```python
from build123d import *

# Parameters (mm, degrees)
SKETCH_1_R      = 1.75
SKETCH_1_R_2    = 1.55
SKETCH_1_W      = 10.25
SKETCH_1_H      = 4.9
EXTRUDE_1_DEPTH = 4
FILLET_1_R      = 1


with BuildPart() as part:
    # 草图1 → 凸台-拉伸1 (new body)
    with BuildSketch(Plane.XY):
        Polygon((-17.225, -19.5), (17.225, -19.5), (17.225, 19.5), (-14.225, 19.5), (-24.725, 19.5), (-24.725, 10.25), (-23.475, 9), (-23.475, 1), (-24.725, -0.25), (-24.725, -8), align=None)
        with BuildLine():
            Line((-5.775, -15.45), (-9.775, -15.45))
            ThreePointArc((-9.775, -15.45), (-10.825, -16.5), (-11.875, -15.45))
            Line((-11.875, -15.45), (-11.875, -12.4))
            ThreePointArc((-11.875, -12.4), (-10.825, -11.35), (-9.775, -12.4))
            Line((-9.775, -12.4), (-5.775, -12.4))
            ThreePointArc((-5.775, -12.4), (-4.725, -11.35), (-3.675, -12.4))
            Line((-3.675, -12.4), (-3.675, -15.45))
            ThreePointArc((-3.675, -15.45), (-4.725, -16.5), (-5.775, -15.45))
        make_face(mode=Mode.SUBTRACT)
        with Locations((-15.725, -7.5)):
            Circle(SKETCH_1_R, mode=Mode.SUBTRACT)
        with Locations((-21.225, -4)):
            Circle(SKETCH_1_R_2, mode=Mode.SUBTRACT)
        Polygon((-3.025, -8.4), (-12.225, -8.4), (-12.725, -8.4), (-12.725, -3.5), (-12.225, -3.5), (-3.025, -3.5), align=None, mode=Mode.SUBTRACT)
        with BuildLine():
            ThreePointArc((6.225, -15.45), (5.175, -16.5), (4.125, -15.45))
            Line((4.125, -15.45), (4.125, -12.4))
            ThreePointArc((4.125, -12.4), (5.175, -11.35), (6.225, -12.4))
            Line((6.225, -12.4), (10.225, -12.4))
            ThreePointArc((10.225, -12.4), (11.275, -11.35), (12.325, -12.4))
            Line((12.325, -12.4), (12.325, -15.45))
            ThreePointArc((12.325, -15.45), (11.275, -16.5), (10.225, -15.45))
            Line((10.225, -15.45), (6.225, -15.45))
        make_face(mode=Mode.SUBTRACT)
        with Locations((7.1, -5.95)):
            Rectangle(SKETCH_1_W, SKETCH_1_H, mode=Mode.SUBTRACT)
        with Locations((-15.725, 7.5)):
            Circle(SKETCH_1_R, mode=Mode.SUBTRACT)
        with Locations((-7.775, 0)):
            Circle(SKETCH_1_R_2, mode=Mode.SUBTRACT)
        Polygon((-12.225, 8.4), (-3.025, 8.4), (-3.025, 3.5), (-12.225, 3.5), (-12.725, 3.5), (-12.725, 8.4), align=None, mode=Mode.SUBTRACT)
        with Locations((-21.225, 14)):
            Circle(SKETCH_1_R_2, mode=Mode.SUBTRACT)
        with BuildLine():
            Line((-5.775, 12.4), (-9.775, 12.4))
            ThreePointArc((-9.775, 12.4), (-10.825, 11.35), (-11.875, 12.4))
            Line((-11.875, 12.4), (-11.875, 15.45))
            ThreePointArc((-11.875, 15.45), (-10.825, 16.5), (-9.775, 15.45))
            Line((-9.775, 15.45), (-5.775, 15.45))
            ThreePointArc((-5.775, 15.45), (-4.725, 16.5), (-3.675, 15.45))
            Line((-3.675, 15.45), (-3.675, 12.4))
            ThreePointArc((-3.675, 12.4), (-4.725, 11.35), (-5.775, 12.4))
        make_face(mode=Mode.SUBTRACT)
        with Locations((6.225, 0)):
            Circle(SKETCH_1_R_2, mode=Mode.SUBTRACT)
        with Locations((7.1, 5.95)):
            Rectangle(SKETCH_1_W, SKETCH_1_H, mode=Mode.SUBTRACT)
        with BuildLine():
            Line((10.225, 12.4), (6.225, 12.4))
            ThreePointArc((6.225, 12.4), (5.175, 11.35), (4.125, 12.4))
            Line((4.125, 12.4), (4.125, 15.45))
            ThreePointArc((4.125, 15.45), (5.175, 16.5), (6.225, 15.45))
            Line((6.225, 15.45), (10.225, 15.45))
            ThreePointArc((10.225, 15.45), (11.275, 16.5), (12.325, 15.45))
            Line((12.325, 15.45), (12.325, 12.4))
            ThreePointArc((12.325, 12.4), (11.275, 11.35), (10.225, 12.4))
        make_face(mode=Mode.SUBTRACT)
    extrude(amount=EXTRUDE_1_DEPTH)

    # 圆角1
    fillet_1_edges = [part.edges().sort_by_distance(p)[0] for p in [
        (-23.475, 1, 2),
        (-23.475, 9, 2),
        (-24.725, 10.25, 2),
        (-24.725, 19.5, 2),
        (17.225, 19.5, 2),
        (17.225, -19.5, 2),
        (-17.225, -19.5, 2),
        (-24.725, -8, 2),
        (-24.725, -0.25, 2),
        (-3.025, -8.4, 2),
        (-3.025, -3.5, 2),
        (-12.725, -3.5, 2),
        (-12.725, -8.4, 2),
        (-3.025, 3.5, 2),
        (-3.025, 8.4, 2),
        (-12.725, 8.4, 2),
        (-12.725, 3.5, 2),
        (12.225, 8.4, 2),
        (1.975, 8.4, 2),
        (1.975, 3.5, 2),
        (12.225, 3.5, 2),
        (1.975, -8.4, 2),
        (12.225, -8.4, 2),
        (12.225, -3.5, 2),
        (1.975, -3.5, 2),
    ]]
    fillet(fillet_1_edges, radius=FILLET_1_R)


solid = part.part
```
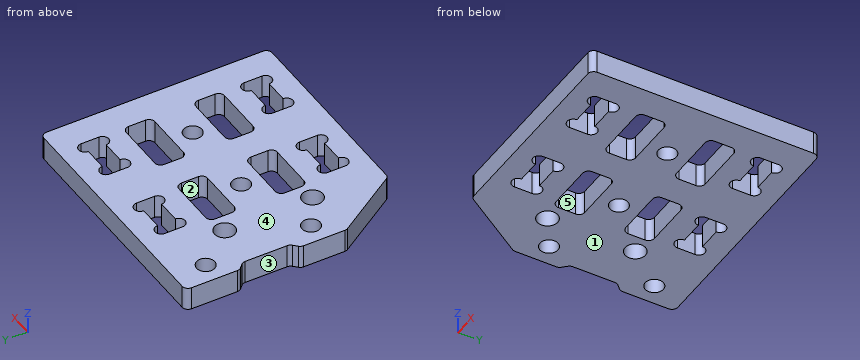
Can you work these out from the model? Positions are in its coordinate system, mm. Face numbers are marked on the shaded views. A direction names the side the tool comes from. Coordinates: 2 decimals unless noted, no trailing zeros. Write each loop counter-clockwise with the first axis right and the second up, starting at its lowest first coordinate (ties: lowest second). Pieces come first, ordered by that corner, then holes. Notation, with made-up numbers: (5.25, -30.75) - (19.25, -30.75) arc R20 ccw to (19.25, -6.75) - close; hole circle Ø9 at (61, 40). An arc over 180 degrees is marked (long way). Return JSON: item names as keys, results as strings.
Q1. Thinking about a two-plate mould opening in Y: for the marked faces 1 and 2, which applies, +Y half, -Y half, draft (parallel to the pull), parting line (faces both ways), or undercut?
Computed values:
{"face 1": "draft", "face 2": "undercut"}
Q2. I'm going to push flat-ended pins straight in: pin 1 Ø1.2 at (y, z) = (4.5, 2.5) entering from -X (3 decimals); pin 2 Ø4 at (x, y) = (-11.5, 9) entering from -Z; pin 3 Ø2 at (x, y) = (10, 13.5) entering from -Z. Where does each tip first touch, or does it pass through?
Computed values:
{"pin 1": "stops at x = -23.475", "pin 2": "stops at z = 0", "pin 3": "passes through"}
Q3. If we section it at A-A (y = -4): Please give me the cut outline in (x, z) (3 decimals), then the cut area to 3 significant figures.
Computed values:
{"outline": "(-24.725, 0) - (-22.775, 0) - (-22.775, 4) - (-24.725, 4) - close; (-19.675, 0) - (-12.591, 0) - (-12.591, 4) - (-19.675, 4) - close; (-3.159, 0) - (2.109, 0) - (2.109, 4) - (-3.159, 4) - close; (12.091, 0) - (17.225, 0) - (17.225, 4) - (12.091, 4) - close", "area": "77.7 mm2"}
Q4. On a 3-axis mill with a long thin cutter (end or side, diameter ignored), from which of +Z, -Z, +X, -X, +Y, -Y can I reach the whole of each face in a straight line? I mean the marked faces 3, 4 and 5. Say none if no direction works.
Computed values:
{"face 3": "+Z, -Z, -X", "face 4": "+Z, +X, -X, +Y, -Y", "face 5": "+Z, -Z"}
Q5. Please list where these lines run through material, in increasing order: L1, parallel to Y at x = 9, z = 2; L2, parallel to X at y = 5, z = 3.7 (3 decimals); L3, parallel to X at y = 4, z = 0.4 (3 decimals). Write a range as from..to.
Computed values:
{"L1": "y = -19.5..-15.45, -12.4..-8.4, -3.5..3.5, 8.4..12.4, 15.45..19.5", "L2": "x = -23.475..-12.725, -3.025..1.975, 12.225..17.225", "L3": "x = -23.475..-12.591, -3.159..2.109, 12.091..17.225"}
Q6. If we section it at C-C (y = 14.5): Please give me the cut outline in (x, z) (3 decimals), then the cut area to 3 significant figures.
Computed values:
{"outline": "(-24.725, 0) - (-22.692, 0) - (-22.692, 4) - (-24.725, 4) - close; (-19.758, 0) - (-11.875, 0) - (-11.875, 4) - (-19.758, 4) - close; (-3.675, 0) - (4.125, 0) - (4.125, 4) - (-3.675, 4) - close; (12.325, 0) - (17.225, 0) - (17.225, 4) - (12.325, 4) - close", "area": "90.5 mm2"}
Q7. If we section it at B-B (z = 3.4): Count the separate pieces of the cut face and the enclosed holes in it, then the cut area to 3 significant figures.
Computed values:
{"separate pieces": "1", "enclosed holes": "14", "area": "1,210 mm2"}
